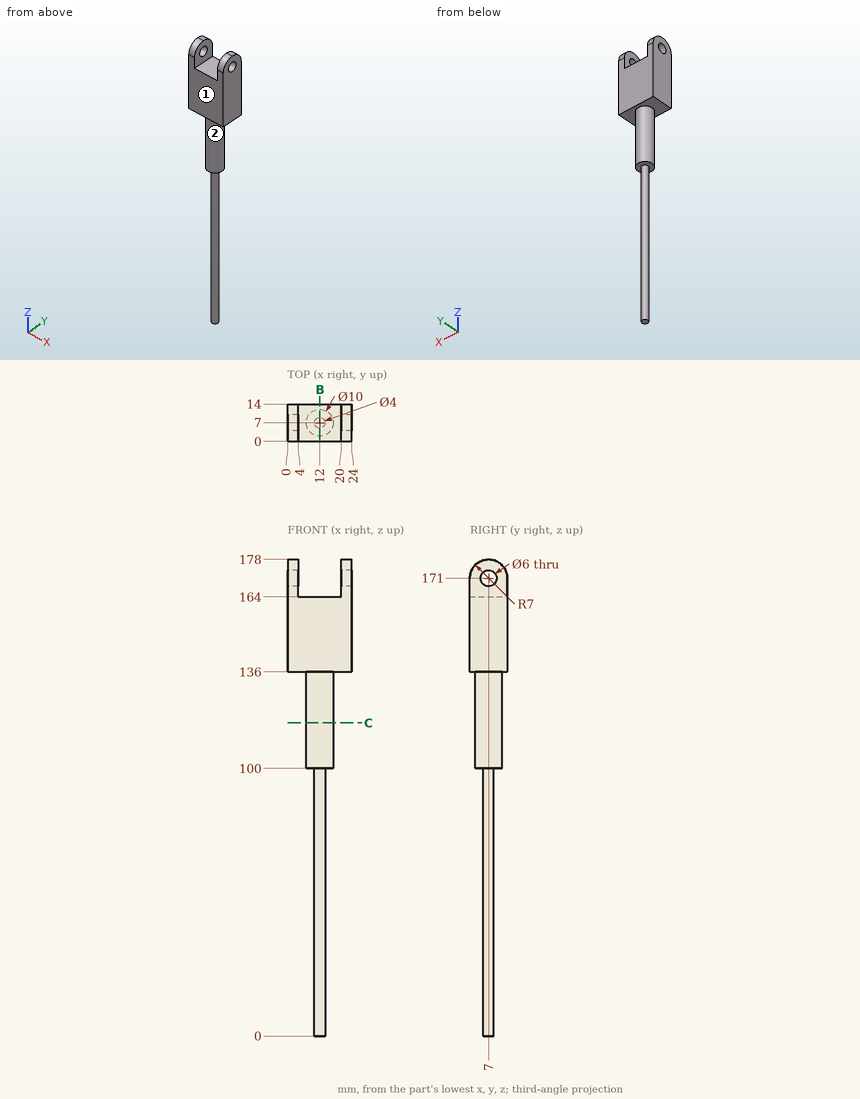
Here's the drawing with two shaded views (mm, measured from the low corner). I have some questions. A direction names the side the tool comes from. Round coordinates to 2 decimals unless told otherwise and drop trailing zeros. Loops run counter-clockwise (first coordinate to the right, second up) from the corner with the lowest first, then second, coordinate; pieces in that order, holes last. Notation, with made-up numbers: (69.5, 42) - (105.5, 42) arc R29 cw to (105.5, 62) - close; hole circle Ø10 at (-29, -2). An arc over 180 degrees is marked (long way). Use CSV: the item, a comma, the result in double quotes.
Item 1: For the marked faces 1 and 2, which set-ups out of +Z, -Z, +X, -X, +Y, -Y let a thin tool reach every point of the face, with its end or its side?
Here are the results:
face 1,"+Z, -Z, +X, -X, -Y"
face 2,"-Z"
Item 2: Will these pins go through, and if not, where does the flat tip stop? pin 1 (4 mm diameter, centred on x = 18.5, z = 101, fed in from -Y); pin 2 (8 mm diameter, centred on x = 10, y = 5, fed in from -Z); pin 3 (3 mm diameter, centred on x = 21, y = 3, fed in from -Z); pin 4 (3 mm diameter, centred on x = 6.5, y = 6, fed in from -Z).
Here are the results:
pin 1,"stops at y = 4.82"
pin 2,"stops at z = 0"
pin 3,"stops at z = 136"
pin 4,"stops at z = 100"
Item 3: If we section it at C-C on z = 117: List the corners of the cut face in (x, y) for me.
Here are the results:
outline,"circle Ø10 at (12, 7)"
Item 4: I need wall thicknesses on L1, parallel to Y at x = 2.05, z = 171; L2, parallel to Z at x = 1.4, y = 7; L3, parallel to Y at x = 12, z = 131. Which ranges of each line are inside material? Lowest first, please. Write a range as [from, to].
Here are the results:
L1,"y = [0, 4], [10, 14]"
L2,"z = [136, 168], [174, 178]"
L3,"y = [2, 12]"
Item 5: If we section it at B-B on x = 12: List the corners of the cut face in (y, z) for me, then the cut area to 3 significant figures.
Here are the results:
outline,"(0, 136) - (2, 136) - (2, 100) - (5, 100) - (5, 0) - (9, 0) - (9, 100) - (12, 100) - (12, 136) - (14, 136) - (14, 164) - (0, 164) - close"
area,"1,150 mm²"
